The listing builds one solid part. Answer for the finished solid, in the listing's coordinates (mm). A direction names the side the tool comes from. Give positions to 0.01 mm unless a question says otherwise; leave off trailing zeros. Answer as a JSON object with one key per item and string values. Group by question number.
Autodesk Fusion 360 part; units mm, degrees
sketch "Sketch1" plane through (0, 0, 0) normal (0, 0, 1) x (1, 0, 0)
  line L0 (0, 0) -> (285, 0)
  line L1 (285, 0) -> (285, 50)
  line L2 (285, 50) -> (0, 50)
  line L3 (0, 50) -> (0, 0)
  line L4 (90.5213, 50) -> (225.5213, 50)
  line L5 (225.5213, 50) -> (225.5213, 75)
  line L6 (225.5213, 75) -> (90.5213, 75)
  line L7 (90.5213, 75) -> (90.5213, 50)
  line L8 (216.9969, 0) -> (193.0469, 0)
  line L9 (202.6853, -0.0546) -> (207.3953, -0.0546)
  line L10 (193.0469, 0) -> (205.0617, 15.8707)
  line L11 (205.0438, 15.8707) -> (216.9969, 0)
  circle A0 centre (140.3583, 38.3038) radius 18.9
  circle A1 centre (102.5213, 63.5005) radius 3.5
  circle A2 centre (118.2718, 63.2499) radius 2.25
  line L12 (111.8584, 9.8039) -> (168.8584, 9.8039)
  line L13 (168.8584, 9.8039) -> (168.8584, 66.8039)
  line L14 (168.8584, 66.8039) -> (111.8584, 66.8039)
  line L15 (111.8584, 66.8039) -> (111.8584, 9.8039)
  line L16 (14.2106, -0.0951) -> (-24.7294, -0.0951)
  line L17 (-24.7294, -0.0951) -> (-10.5221, 12.6845)
  line L18 (-10.5221, 12.6845) -> (-0.0196, 12.6845)
  line L19 (-0.0196, 12.6845) -> (14.2106, -0.0951)
  dimension "d1" = 285
  dimension "d2" = 50
  dimension "d7" = 135
  dimension "d8" = 25
  dimension "d36" = 23.95
  dimension "d37" = 4.71
  dimension "d41" = 37.8
  dimension "d42" = 7
  dimension "d43" = 4.5
  dimension "d45" = 57
  dimension "d46" = 57
  dimension "d52" = 38.94
extrude "Extrude2" add sketch "Sketch1" along normal blind 6 contours L0 L1 L2 L3 L4 L10 L11 L12 L13 L15 L19 | L2 L4 L5 L6 L7 L13 L14 L15 | L2 L4 A0 L12 L13 L15 | L2 L4 A0 L13 L14 L15 | L2 L4 A0 | L2 L4 A0 | A1 | A2
chamfer "Chamfer9" distance 10 angle 45 5 edges at (285, 0, 3) (285, 50, 3) (225.5213, 50, 3) (90.5213, 50, 3) (0, 50, 3)
fillet "Fillet19" radius 4 17 edges at (216.9969, 0, 3) (193.0469, 0, 3) (205.0527, 15.8588, 3) (0, 12.667, 3) (14.1047, 0, 3) (0, 40, 3) (10, 50, 3) (90.5213, 60, 3) (80.5213, 50, 3) (225.5213, 60, 3) (235.5213, 50, 3) (275, 50, 3) (285, 40, 3) (285, 10, 3) (275, 0, 3) (90.5213, 75, 3) (225.5213, 75, 3)
equation "DBigHull = 3.78 cm"
equation "AvstandFraLangKantTilBigHull = 12.32 cm"
equation "motorfront = 56 mm"
equation "d41 = DBigHull"
equation "NEM23 = 57 mm"
equation "d45 = NEM23"
equation "d46 = NEM23"
Item 1: Flat-ended cylindrical pins translate along their axes: P1, Ø2, axis at y = 48, z = 5, coming from the +X side; P2, Ø10, axis at x = 105, y = 20.5, coming from the -Z side; P3, Ø2, axis at x = 64.5, z = 1, coming from the +Y side. Find the tip coordinate at first contact, or state that the pin passes through.
Item 2: A tool of negligible diameter and unlimited length cuts with its end or side. For faces 4 (the flat face through (225.521, 66, 3)), 5 (the flat face through (46, 50, 3)), 6 (the flat face through (211.965, 6.681, 2.958)), from which of +Z, -Z, +X, -X, +Y, -Y can it reach the whole face along a straight path? Write none if from no direction.
Item 3: Determine the mould class of faces 1 (the flat face through (90.521, 66, 3)), 2 (the cylindrical face through (205.1, 13.22, 3.04)), 3 (the flat face through (280, 5, 3)) for opening direction X: released by +X, released by -X, zero draft, split by the parting line, or undercut.
Item 4: Consider probe 1 along Y at (x, z) = (63.5, 3.65); probe 2 along X at (y, z) = (64.5, 1); probe 3 along Y at (x, z) = (194, 4.4). Determine where each line is inside the solid, lowest interval first. Write a range as from..to.
Values found:
{
 "1": {"P1": "stops at x = 278", "P2": "stops at z = 0", "P3": "stops at y = 50"},
 "2": {"face 4": "+Z, -Z, +X, +Y", "face 5": "+Z, -Z, -X, +Y", "face 6": "+Z, -Z, -Y"},
 "3": {"face 1": "released by -X", "face 2": "undercut", "face 3": "released by +X"},
 "4": {"probe 1": "y = 0..50", "probe 2": "x = 90.52..225.52", "probe 3": "y = 1.29..75"}
}
